Input: part model. Units: mm. Frame: model coordinates. Round coordinates to 2 decimals unless told otherwise and drop trailing zeros. Order: outer loops, then holes, each group sorted by start corner. A loop starts at its lowest first (then second) coordinate and runs counter-clockwise, first axis right, second up. Notation, with made-up numbers: M -6.75,15 L 33.25,15 A16 ccw 33.25,39 Z; hole C 61.25,-31.75 d8. An arc over 180 degrees is marked long. One line per question, with ' | ' between items.
```python
from build123d import *

# Parameters (mm, degrees)
BASE_FLANGE1_DEPTH  = 0.7
BREAK_CORNER1_START = -0.7
BREAK_CORNER1_DEPTH = 0.7


# Read off the part's stored shape, not the designer's step: Break-Corner1
# Sheet-metal steps are written as plain solids
with BuildPart() as part:
    # Sketch1 → Base-Flange1 (new body)
    with BuildSketch(Plane.XY):
        Polygon((0, 0), (0, 35), (-35, 0), align=None)
    extrude(amount=-BASE_FLANGE1_DEPTH)

    # Break-Corner1 outline → Break-Corner1 (cut)
    with BuildSketch(Plane.XY.offset(BREAK_CORNER1_START)):
        with BuildLine():
            ThreePointArc((-28.964466094, 0), (-31.274164925, 1.543291419), (-30.732233047, 4.267766953))
            Line((-30.732233047, 4.267766953), (-35, 0))
            Line((-35, 0), (-28.964466094, 0))
        make_face()
        with BuildLine():
            Line((0, 35), (-4.267766953, 30.732233047))
            ThreePointArc((-4.267766953, 30.732233047), (-1.543291419, 31.274164925), (0, 28.964466094))
            Line((0, 28.964466094), (0, 35))
        make_face()
        with BuildLine():
            ThreePointArc((0, 2.5), (-0.732233047, 0.732233047), (-2.5, 0))
            Line((-2.5, 0), (0, 0))
            Line((0, 0), (0, 2.5))
        make_face()
    extrude(amount=BREAK_CORNER1_DEPTH, mode=Mode.SUBTRACT)


solid = part.part
```
Item 1: Line query: line 1 along Y through (x, z) = (-12.5, -0.4); line 2 along Y through (x, z) = (-6, -0.6); line 3 along X through (y, z) = (3, -0.4). Output: solid intervals per line, ascending. Write a range as from..to.
Report:
line 1: 0..22.5 | line 2: 0..29 | line 3: -31.41..0
Item 2: Section query A-A, the plane z = -0.45. Return loops of the section in (x, y), plus the area to 3 significant figures.
Report:
outline: M -30.73,4.27 A2.5 ccw -28.96,0 L -2.5,0 A2.5 ccw 0,2.5 L 0,28.96 A2.5 ccw -4.27,30.73 Z | area: 596 mm²
Item 3: Section query B-B, the plane x = -8.5. Return loops of the section in (y, z), plus the area to 4 significant figures.
Report:
outline: M 0,-0.7 L 26.5,-0.7 L 26.5,0 L 0,0 Z | area: 18.55 mm²
Item 4: Section query C-C, the plane y = 16.5. Return loops of the section in (x, z), plus the area to 4 significant figures.
Report:
outline: M -18.5,-0.7 L 0,-0.7 L 0,0 L -18.5,0 Z | area: 12.95 mm²
